Check sheet for the modelled part. Datum: model origin and axes. Units: mm. A direction names the side the tool comes from. Coordinates: 2 decimals unless noted, no trailing zeros. Write each loop counter-clockwise with the first axis right and the second up, starting at its lowest first coordinate (ties: lowest second). Pieces come first, ordered by that corner, then holes. Notation, with made-up numbers: (-8, 81) - (42, 81) arc R33 ccw to (42, 115) - close; hole circle Ø5 at (49.25, 15). An arc over 180 degrees is marked (long way). Write each question's results on one line, items separated by ' | '.
from build123d import *

# Parameters (mm, degrees)
ESQUISSE3_R             = 12.5
ESQUISSE3_W             = 25
ESQUISSE3_H             = 12.5
BOSS_EXTRU_2_DEPTH      = 20
ESQUISSE4_R             = 7.5
ENL_V_MAT_EXTRU_1_DEPTH = 41.620192023
TROU_TARAUD_M51_D       = 4.2
TROU_TARAUD_M51_DEPTH   = 5
TROU_TARAUD_M51_TIP     = 1.2618073


with BuildPart() as part:
    # Esquisse3 → Boss.-Extru.2 (new body)
    with BuildSketch(Plane(origin=(0, 0, 0), x_dir=(0, 0, -1), z_dir=(1, 0, 0))):
        with Locations((12.5, 12.5)):
            Circle(ESQUISSE3_R)
        with Locations((12.5, 6.25)):
            Rectangle(ESQUISSE3_W, ESQUISSE3_H)
    extrude(amount=BOSS_EXTRU_2_DEPTH)

    # Esquisse4 → Enlèv. mat.-Extru.1 (cut, through all)
    with BuildSketch(Plane.ZY):
        with Locations((-12.5, 12.5)):
            Circle(ESQUISSE4_R)
    extrude(amount=-ENL_V_MAT_EXTRU_1_DEPTH, mode=Mode.SUBTRACT)

    # Trou taraudé M51
    with Locations(Plane(origin=(10, 0, -5), x_dir=(0, 0, -1), z_dir=(0, -1, 0))):
        with Locations((0, 0), (15, 0)):
            Hole(TROU_TARAUD_M51_D / 2, depth=TROU_TARAUD_M51_DEPTH)
            with Locations((0, 0, -(TROU_TARAUD_M51_DEPTH + TROU_TARAUD_M51_TIP / 2))):  # 118° drill point
                Cone(0, TROU_TARAUD_M51_D / 2, TROU_TARAUD_M51_TIP, mode=Mode.SUBTRACT)


solid = part.part
1. Go/stop test with flat-tipped pins: pin 1 (5.5 mm diameter, centred on x = 10, z = -20, fed in from +Y); pin 2 (8 mm diameter, centred on x = 5, z = -4, fed in from +Y); pin 3 (4 mm diameter, centred on x = 7, y = 19, fed in from +Z). Record where each tip stops, or that it passes through.
Values follow:
pin 1: stops at y = 24.06 | pin 2: stops at y = 24.16 | pin 3: stops at z = -0.84
2. Sectioned sample at D-D (y = 17.75). Record the cut outline in (x, z), then the cut area to 3 significant figures.
Values follow:
outline: (0, -23.84) - (20, -23.84) - (20, -17.86) - (0, -17.86) - close; (0, -7.14) - (20, -7.14) - (20, -1.16) - (0, -1.16) - close | area: 240 mm^2
3. Sectioned sample at B-B (y = 2.25). Record the cut outline in (x, z), then the cut area to 3 significant figures.
Values follow:
outline: (0, -25) - (20, -25) - (20, 0) - (0, 0) - close; hole circle Ø4.2 at (10, -20); hole circle Ø4.2 at (10, -5) | area: 472 mm^2
4. Sectioned sample at A-A (z = -12.5). Record the cut outline in (x, y), then the cut area to 3 significant figures.
Values follow:
outline: (0, 0) - (20, 0) - (20, 5) - (0, 5) - close; (0, 20) - (20, 20) - (20, 25) - (0, 25) - close | area: 200 mm^2
5. Draft check along X on faces 1 (the flat face through (20, 7, -18)), 2 (the cylindrical face through (9.86, 24.997, -12.775)), 3 (the flat face through (0, 7, -18)), 4 (the conical face through (10.25, 6.04, -19.73)). Enter one of: pulls with the +X half, pulls with the -X half, needs draft (parallel to the pull), parting line crosses it, or undercut.
Values follow:
face 1: pulls with the +X half | face 2: needs draft | face 3: pulls with the -X half | face 4: undercut
6. Access from +Z, -Z, +X, -X, +Y, -Y to the whole of each face (thin tool, end or side, straight path). Record for faces 5 (the flat face through (10, 6, 0)), 6 (the cylindrical face through (12.082, 2.535, -5.273)).
Values follow:
face 5: +Z, +X, -X, +Y, -Y | face 6: -Y
7. Sectioned sample at C-C (x = 14.75). Record the cut outline in (y, z), then the cut area to 3 significant figures.
Values follow:
outline: (0, -25) - (12.5, -25) arc R12.5 ccw to (12.5, 0) - (0, 0) - close; hole circle Ø15 at (12.5, -12.5) | area: 381 mm^2
8. Material ranges on L1, parallel to Z at x = 10, y = 3.7; L2, parallel to Y at x = 9, z = -12.5; L3, parallel to X at y = 1.25, z = -20, recorded low to high. Write a range as [from, to].
Values follow:
L1: z = [-25, -22.1], [-17.9, -7.1], [-2.9, 0] | L2: y = [0, 5], [20, 25] | L3: x = [0, 7.9], [12.1, 20]
